Design review of the part built by this model. Coordinates are the model's own, in mm. Face numbers are marked on the shaded views. A direction names the side the tool comes from. Give positions to 0.01 mm unless a question says otherwise; leave off trailing zeros. Loops run counter-clockwise (first coordinate to the right, second up) from the corner with the lowest first, then second, coordinate; pieces in that order, holes last. Notation, with made-up numbers: M 20,66.25 L 54,66.25 A15 cw 54,73.25 Z; hole C -33,76 d1. An arc over 180 degrees is marked long. Use one line per item in the form item = value. Start each with the question number.
from build123d import *

# Parameters (mm, degrees)
BOSS_EXTRUDE1_DEPTH = 6.35
BOSS_EXTRUDE2_DEPTH = 60.325
SKETCH2_W           = 6.35
SKETCH2_H           = 76.2
BOSS_EXTRUDE3_DEPTH = 12.7
CUT_EXTRUDE2_REACH  = 87.784
CUT_EXTRUDE3_REACH  = 87.784
SKETCH4_3_R         = 3.96875
SKETCH7_W           = 36.5125
SKETCH7_H           = 3.175
BOSS_EXTRUDE5_DEPTH = 12.7
CHAMFER6_SIZE       = 6.35


with BuildPart() as part:
    # Sketch1 → Boss-Extrude1 (new body)
    with BuildSketch(Plane(origin=(0, 0, 0), x_dir=(1, 0, 0), z_dir=(0, 1, 0))):
        Polygon((19.05, 34.925), (19.05, 38.1), (-23.8125, 38.1), (-23.8125, -38.1), (19.05, -38.1), (19.05, -34.925), (-17.4625, -34.925), (-17.4625, 34.925), align=None)
    extrude(amount=BOSS_EXTRUDE1_DEPTH)

    # Sketch1<4> → Boss-Extrude2 (add)
    with BuildSketch(Plane(origin=(0, 0, 0), x_dir=(1, 0, 0), z_dir=(0, 1, 0))):
        Polygon((23.8125, 38.1), (19.05, 38.1), (19.05, 34.925), (19.05, -34.925), (19.05, -38.1), (23.8125, -38.1), align=None)
    extrude(amount=BOSS_EXTRUDE2_DEPTH)

    # Sketch2 → Boss-Extrude3 (add)
    with BuildSketch(Plane(origin=(0, 6.35, 0), x_dir=(1, 0, 0), z_dir=(0, 1, 0))):
        with Locations((-20.6375, 0)):
            Rectangle(SKETCH2_W, SKETCH2_H)
    extrude(amount=BOSS_EXTRUDE3_DEPTH)

    # Sketch4 → Cut-Extrude2 (cut, up to next)
    with BuildSketch(Plane(origin=(23.8125, 0, 0), x_dir=(0, 0, -1), z_dir=(1, 0, 0)), mode=Mode.PRIVATE) as cut_extrude2_sk1:
        with BuildLine():
            Line((-38.1, 60.325), (-38.1, 31.75))
            Line((-38.1, 31.75), (-12.7, 50.8))
            ThreePointArc((-12.7, 50.8), (-7.9375, 57.679166667), (0, 60.325))
            Line((0, 60.325), (-38.1, 60.325))
        make_face()
    cut_extrude2_tool1 = extrude(cut_extrude2_sk1.sketch, amount=-CUT_EXTRUDE2_REACH, mode=Mode.PRIVATE) & part.part
    # Sketch4 → Cut-Extrude2 (cut, up to next)
    with BuildSketch(Plane(origin=(23.8125, 0, 0), x_dir=(0, 0, -1), z_dir=(1, 0, 0)), mode=Mode.PRIVATE) as cut_extrude2_sk2:
        with BuildLine():
            Line((38.1, 60.325), (0, 60.325))
            ThreePointArc((0, 60.325), (7.9375, 57.679166667), (12.7, 50.8))
            Line((12.7, 50.8), (38.1, 31.75))
            Line((38.1, 31.75), (38.1, 60.325))
        make_face()
    cut_extrude2_tool2 = extrude(cut_extrude2_sk2.sketch, amount=-CUT_EXTRUDE2_REACH, mode=Mode.PRIVATE) & part.part
    add(cut_extrude2_tool1.solids().sort_by_distance((23.8125, 50.488362, 26.421388))[0], mode=Mode.SUBTRACT)
    add(cut_extrude2_tool2.solids().sort_by_distance((23.8125, 50.488362, -26.421388))[0], mode=Mode.SUBTRACT)

    # Sketch4<3> → Cut-Extrude3 (cut, up to next)
    with BuildSketch(Plane(origin=(23.8125, 0, 0), x_dir=(0, 0, -1), z_dir=(1, 0, 0)), mode=Mode.PRIVATE) as cut_extrude3_sk1:
        with Locations((0, 50.8)):
            Circle(SKETCH4_3_R)
    cut_extrude3_tool1 = extrude(cut_extrude3_sk1.sketch, amount=-CUT_EXTRUDE3_REACH, mode=Mode.PRIVATE) & part.part
    add(cut_extrude3_tool1.solids().sort_by_distance((23.8125, 50.8, 0))[0], mode=Mode.SUBTRACT)

    # Sketch7 → Boss-Extrude5 (add)
    with BuildSketch(Plane(origin=(0, 6.35, 0), x_dir=(1, 0, 0), z_dir=(0, 1, 0))):
        with Locations((0.79375, 36.5125)):
            Rectangle(SKETCH7_W, SKETCH7_H)
        with Locations((0.79375, -36.5125)):
            Rectangle(SKETCH7_W, SKETCH7_H)
    extrude(amount=BOSS_EXTRUDE5_DEPTH)

    # Chamfer6
    chamfer6_edges = [part.edges().sort_by_distance(p)[0] for p in [
        (-17.4625, 9.525, 34.925),
        (19.05, 9.525, 34.925),
        (19.05, 9.525, -34.925),
        (-17.4625, 9.525, -34.925),
    ]]
    chamfer(chamfer6_edges, length=CHAMFER6_SIZE)


solid = part.part
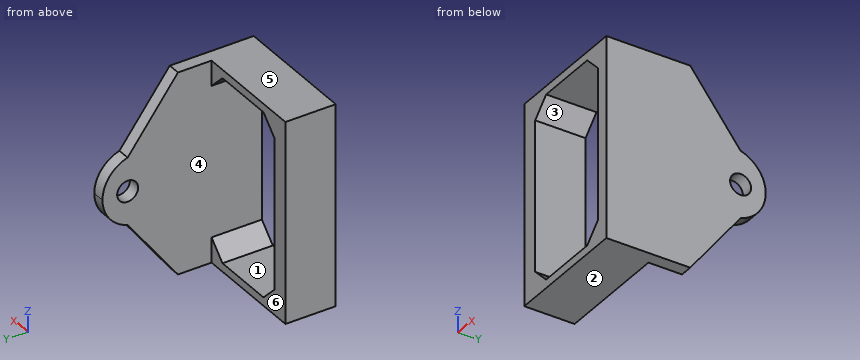
Q1. Clearance check with a flat-ended pin moving along its axis: pin 1 Ø5 at (x, z) = (15.5, 13) entering from +Y. State where the tip first meets the part, or that it passes through.
Q2. Take a section at A-A on z = -19.5. Give the boundary of the cut face in (x, y), plus the area to 3 significant figures.
Q3. Wall thickness on probe 1 along X at (y, z) = (13, -24.5); probe 2 along Y at (x, z) = (21.6, 0) (3 decimals); probe 3 along Z at (x, y) = (-8, 9.5) (3 decimals): over which ranges is each line inside the solid? List them lowest first.
Q4. Take a section at C-C on y = 34. Give the boundary of the cut face in (x, z), plus the area to 3 significant figures.
Q5. For the marked faces 1 and 2, list the 3-axis set-ups (+Z, -Z, +X, -X, +Y, -Y) from which the entire face can be reached by the end or side of a thin tool; tool diameter is ignored.
Q6. The part is to be moulded in two halves that separate along Z. For the marked faces 3, 4, 5 and 6, say which applies: pulls with the +Z half, pulls with the -Z half, needs draft (parallel to the pull), parting line crosses it, or undercut.
Q7. Take a section at B-B on x = 10. Give the boundary of the cut face in (y, z) (3 decimals).
Response values:
q1.pin_1 = through
q2.outline = M -23.81,0 L -17.46,0 L -17.46,19.05 L -23.81,19.05 Z; M 19.05,0 L 23.81,0 L 23.81,45.7 L 19.05,45.7 Z
q2.area = 339 mm^2
q3.probe_1 = -23.81 to -17.46, 19.05 to 23.81
q3.probe_2 = 0 to 46.831, 54.769 to 60.325
q3.probe_3 = -38.1 to -34.925, 34.925 to 38.1
q4.outline = M 19.05,-35.1 L 23.81,-35.1 L 23.81,35.1 L 19.05,35.1 Z
q4.area = 334 mm^2
q5.face_1 = +Y, -Y
q5.face_2 = -Z, +X, -X, +Y, -Y
q6.face_3 = undercut
q6.face_4 = undercut
q6.face_5 = pulls with the +Z half
q6.face_6 = needs draft
q7.outline = M 0,-38.1 L 19.05,-38.1 L 19.05,-34.925 L 0,-34.925 Z; M 0,34.925 L 19.05,34.925 L 19.05,38.1 L 0,38.1 Z
